For this review, take the finished solid that the model builds, in its own axes (mm). A direction names the side the tool comes from. Give positions to 0.01 mm unless a question says otherwise; leave off trailing zeros. Write each loop counter-clockwise with the first axis right and the second up, starting at its lowest first coordinate (ties: lowest second). Pieces come first, ordered by that corner, then holes.
Q1. Machinability: for faces 4 (the flat face through (-13, 9, -57.15)), 5 (the flat face through (-19.05, 9, -64)), 6 (the flat face through (-6.35, 9, -63)), 7 (the flat face through (-13, 15.081, -64)), which of the approach directions +Z, -Z, +X, -X, +Y, -Y give a long, thin tool a straight path to every point of the face, cutting with its end or side? Answer none if there is none.
Q2. For line 1 (Z direction, x = -13.75, y = 2.5); line 2 (Y direction, x = -6.5, z = -54), list the stretches that pass through material, from the lowest coordinate up.
Q3. We need section B-B (z = -66). Write out the cut boundary in (x, y), then the cut area to 3 significant figures.
Q4. We need section C-C (y = 3). Write out the cut boundary in (x, z), then the cut area to 3 significant figures.
Q5. Insertion check: P1, Ø4, axis at y = 8.5, z = -66, coming from the +X side; P2, Ø5, axis at x = -10, y = 12.5, coming from the +Z side; P3, Ø12, axis at x = -10.5, z = -33, coming from the +Y side. Each pin has a flat end and moves straight along its axis. Give the tip position at first contact, or say it passes through.
Q6. We need section A-A (x = -14.5). Write out the cut boundary in (y, z), then the cut area to 3 significant figures.
Q7. We need section D-D (z = -15.5). Write out the cut boundary in (x, y), then the cut area to 3 significant figures.
Q8. Mouldability with a two-part tool opening along X and no side actions: class faces 1 (the flat face through (-13, 2.381, -34)), 2 (the flat face through (-25.4, 1, -34)), 3 (the flat face through (0, 1, -35)) as released by +X, released by -X, zero draft, split by the parting line, or undercut.
Autodesk Inventor part; units mm, degrees
ref_plane "YZ Plane" through (0, 0, 0) normal (1, 0, 0) x (0, 1, 0)
ref_plane "XZ Plane" through (0, 0, 0) normal (0, 1, 0) x (-1, 0, 0)
ref_plane "XY Plane" through (0, 0, 0) normal (0, 0, 1) x (1, 0, 0)
sketch "Sketch1" plane through (0, 0, 0) normal (0, 1, 0) x (-1, 0, 0)
  line L0 (0, 0) -> (25.4, 0)
  line L1 (25.4, 0) -> (25.4, -69.85)
  line L2 (25.4, -69.85) -> (0, -69.85)
  line L3 (0, -69.85) -> (0, 0)
  dimension "d0" = 25.4
  dimension "d1" = 69.85
extrude "Extrusion1" add sketch "Sketch1" along normal blind 2.3813
sketch "Sketch2" plane through (0, 2.3813, 0) normal (0, 1, 0) x (1, 0, 0)
  line L0 (0, 69.85) -> (-25.4, 69.85)
  line L1 (0, 69.85) -> (-6.35, 69.85)
  line L2 (-6.35, 69.85) -> (-19.05, 69.85)
  line L3 (-19.05, 69.85) -> (-19.05, 57.15)
  line L4 (-19.05, 57.15) -> (-6.35, 57.15)
  line L5 (-6.35, 57.15) -> (-6.35, 69.85)
  point P0 (0, 0)
  dimension "d4" = 6.35
  dimension "d5" = 12.7
  dimension "d6" = 12.7
extrude "Extrusion2" add sketch "Sketch2" along normal blind 12.7
properties part number "WaterSensor"
Computed:
1. face 4: +Z, +X, -X, +Y
1. face 5: +Z, -Z, -X, +Y
1. face 6: +Z, -Z, +X, +Y
1. face 7: +Z, -Z, +X, -X, +Y
2. line 1: z = -69.85 to -57.15
2. line 2: y = 0 to 2.38
3. outline: (-25.4, 0) - (0, 0) - (0, 2.38) - (-6.35, 2.38) - (-6.35, 15.08) - (-19.05, 15.08) - (-19.05, 2.38) - (-25.4, 2.38) - close
3. area: 222 mm2
4. outline: (-19.05, -69.85) - (-6.35, -69.85) - (-6.35, -57.15) - (-19.05, -57.15) - close
4. area: 161 mm2
5. P1: stops at x = -6.35
5. P2: stops at z = -57.15
5. P3: stops at y = 2.38
6. outline: (0, -69.85) - (15.08, -69.85) - (15.08, -57.15) - (2.38, -57.15) - (2.38, 0) - (0, 0) - close
6. area: 328 mm2
7. outline: (-25.4, 0) - (0, 0) - (0, 2.38) - (-25.4, 2.38) - close
7. area: 60.5 mm2
8. face 1: zero draft
8. face 2: released by -X
8. face 3: released by +X
